Part model, mm, in its own coordinate system. Face numbers are marked on the shaded views. A direction names the side the tool comes from. Round coordinates to 2 decimals unless told otherwise and drop trailing zeros. Loops run counter-clockwise (first coordinate to the right, second up) from the corner with the lowest first, then second, coordinate; pieces in that order, holes last.
1) 3-axis set-ups, long thin cutter, end or side, ignore diameter. For the marked faces 1, 2 and 3: which of +Z, -Z, +X, -X, +Y, -Y reach the whole face in a straight line?
2) Band-saw the part on C-C, the plane x = 70.5. Write the cut outline in (y, z).
3) Band-saw the part on B-B, the plane y = 0. Write the cut outline in (x, z), then the cut area to 3 significant figures.
4) Band-saw the part on A-A, the plane x = 23.5. Write the cut outline in (y, z).
5) Drop flat-ended pins along their axis: P1, Ø1, axis at y = -12, z = 0.5, coming from the -X side; P2, Ø19, axis at x = 3.5, y = -5.5, coming from the -Z side; P3, Ø4, axis at x = 25, y = 24, coming from the -Z side; P4, Ø6, axis at x = -4.5, y = 5, coming from the +Z side. Give the stop position or say it passes through.
6) Probe line 1 (Y direction, x = -23.5, z = 3.45); line 2 (Y direction, x = -16.25, z = 0); line 3 (Y direction, x = -23.5, z = -1.35). List the from-to ranges inside material, lowest first.
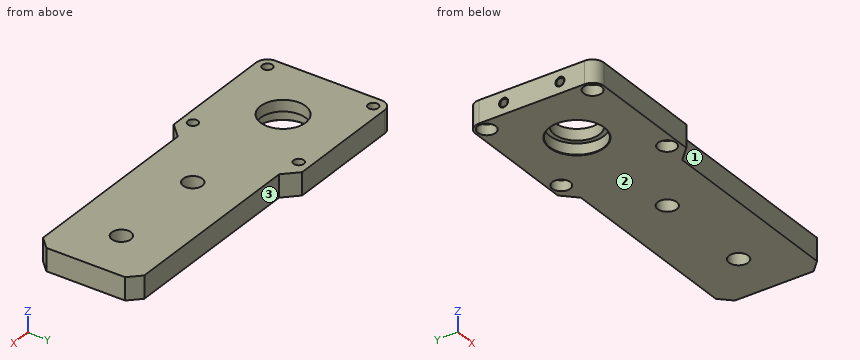
from build123d import *

# Parameters (mm, degrees)
EXTRUDE_1_DEPTH              = 5
SKETCH_6_R                   = 10
CUT_EXTRUDE_1513_DEPTH       = 10
SKETCH_19_R                  = 12
CUT_EXTRUDE_1929_DEPTH       = 5
HOLE_WIZARD_8_5_8_5_1_D      = 8.5
HOLE_WIZARD_1_D              = 4.5
HOLE_WIZARD_1_CBORE_D        = 8
HOLE_WIZARD_1_CBORE_DEPTH    = 4.6
FILLET_1_R                   = 5
CHAMFER_1_SIZE               = 5
CHAMFER_2_SIZE               = 0.2
HOLE_WIZARD_M4_1_D           = 3.3
HOLE_WIZARD_M4_1_DEPTH       = 15.5
HOLE_WIZARD_M4_1_CSINK_D     = 4.05
HOLE_WIZARD_M4_1_CSINK_ANGLE = 120


with BuildPart() as part:
    # 草图1 → 凸台-拉伸1 (new body, symmetric)
    with BuildSketch(Plane.XY):
        Polygon((28.5, 28.5), (-28.5, 28.5), (-28.5, -28.5), (28.5, -28.5), (34.5, -22.5), (124.5, -22.5), (124.5, 22.5), (34.5, 22.5), align=None)
    extrude(amount=EXTRUDE_1_DEPTH, both=True)

    # 草图6 → Cut-Extrude 1513 (cut)
    with BuildSketch(Plane.XY.offset(5)):
        Circle(SKETCH_6_R)
    extrude(amount=-CUT_EXTRUDE_1513_DEPTH, mode=Mode.SUBTRACT)

    # 草图19 → Cut-Extrude 1929 (cut)
    with BuildSketch(Plane(origin=(0, 0, -5), x_dir=(-1, 0, 0), z_dir=(0, 0, -1))):
        Circle(SKETCH_19_R)
    extrude(amount=-CUT_EXTRUDE_1929_DEPTH, mode=Mode.SUBTRACT)

    # Ø8.5 (8.5) 直径孔1 (through all)
    with Locations(Plane.XY.offset(5)):
        with Locations((57, 0), (102, 0)):
            Hole(HOLE_WIZARD_8_5_8_5_1_D / 2)

    # 打孔尺寸(%根据)内六角圆柱头螺钉的类型1 (through all)
    with Locations(Plane(origin=(0, 0, -5), x_dir=(-1, 0, 0), z_dir=(0, 0, -1))):
        with Locations((-23.5, 23.5), (23.5, 23.5), (23.5, -23.5), (-23.5, -23.5)):
            CounterBoreHole(HOLE_WIZARD_1_D / 2, HOLE_WIZARD_1_CBORE_D / 2, HOLE_WIZARD_1_CBORE_DEPTH)

    # 圆角1
    fillet_1_edges = [part.edges().sort_by_distance(p)[0] for p in [
        (-28.5, -28.5, 0),
        (-28.5, 28.5, 0),
    ]]
    fillet(fillet_1_edges, radius=FILLET_1_R)

    # 倒角1
    chamfer_1_edges = [part.edges().sort_by_distance(p)[0] for p in [
        (124.5, 22.5, 0),
        (124.5, -22.5, 0),
    ]]
    chamfer(chamfer_1_edges, length=CHAMFER_1_SIZE)

    # 倒角2
    chamfer_2_edges = [part.edges().sort_by_distance(p)[0] for p in [
        (12, 0, -5),
    ]]
    chamfer(chamfer_2_edges, length=CHAMFER_2_SIZE)

    # M4 螺纹孔1
    with Locations(Plane.ZY.offset(28.5)):
        with Locations((0, 12.5), (0, -12.5)):
            CounterSinkHole(HOLE_WIZARD_M4_1_D / 2, HOLE_WIZARD_M4_1_CSINK_D / 2, depth=HOLE_WIZARD_M4_1_DEPTH, counter_sink_angle=HOLE_WIZARD_M4_1_CSINK_ANGLE)


solid = part.part
Reported:
1. face 1: +Z, -Z, +X, -Y
1. face 2: -Z, +X, -X, +Y, -Y
1. face 3: +Z, -Z, +X, +Y
2. outline: (-22.5, -5) - (22.5, -5) - (22.5, 5) - (-22.5, 5) - close
3. outline: (-28.5, -5) - (-12.2, -5) - (-12, -4.8) - (-12, 0) - (-10, 0) - (-10, 5) - (-28.5, 5) - close; (10, 0) - (12, 0) - (12, -4.8) - (12.2, -5) - (52.75, -5) - (52.75, 5) - (10, 5) - close; (61.25, -5) - (97.75, -5) - (97.75, 5) - (61.25, 5) - close; (106.25, -5) - (124.5, -5) - (124.5, 5) - (106.25, 5) - close
3. area: 1,140 mm2
4. outline: (-28.5, -5) - (-27.5, -5) - (-27.5, -0.4) - (-25.75, -0.4) - (-25.75, 5) - (-28.5, 5) - close; (-21.25, -0.4) - (-19.5, -0.4) - (-19.5, -5) - (19.5, -5) - (19.5, -0.4) - (21.25, -0.4) - (21.25, 5) - (-21.25, 5) - close; (25.75, -0.4) - (27.5, -0.4) - (27.5, -5) - (28.5, -5) - (28.5, 5) - (25.75, 5) - close
5. P1: stops at x = -13
5. P2: stops at z = -5
5. P3: stops at z = -0.4
5. P4: passes through
6. line 1: y = -28.5 to -25.75, -21.25 to 21.25, 25.75 to 28.5
6. line 2: y = -28.5 to -14.15, -10.85 to 10.85, 14.15 to 28.5
6. line 3: y = -28.5 to -27.5, -19.5 to -13.45, -11.55 to 11.55, 13.45 to 19.5, 27.5 to 28.5
